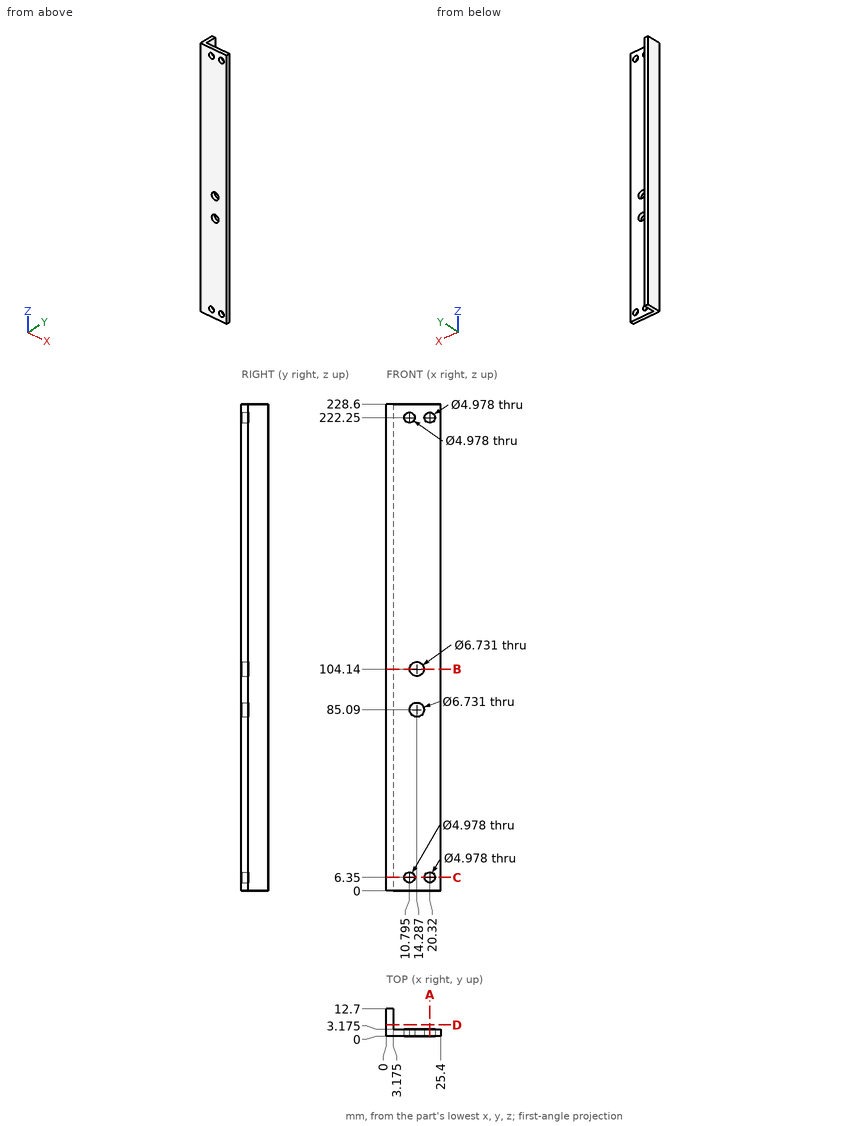
Input: dimensioned drawing with shaded views. Units: mm. Origin: part minimum x, y, z. Coordinates: 2 decimals unless noted, no trailing zeros. Order: outer loops, then holes, each group sorted by start corner. A loop starts at its lowest first (then second) coordinate and runs counter-clockwise, first axis right, second up.
Item 1: Material intervals for line 1 along X through (y, z) = (1.45, 222.25) (1 decimal); line 2 along Z through (x, y) = (20.32, 1.6); line 3 along X through (y, z) = (1.35, 104.14), sorted ascending.
Answer:
line 1: x = 0 to 8.3, 13.3 to 17.8, 22.8 to 25.4
line 2: z = 0 to 3.86, 8.84 to 219.76, 224.74 to 228.6
line 3: x = 0 to 10.92, 17.65 to 25.4
Item 2: Contact query for flat-ended pins moving along their axis: P1, Ø4, axis at x = 10.795, z = 6.35, coming from the +Y side; P2, Ø5, axis at y = 6, z = 109, coming from the +X side (1 decimal); P3, Ø11, axis at x = 14.29, z = 104.14, coming from the +Y side (1 decimal). Output: stop coordinate, or through.
Answer:
P1: passes through
P2: stops at x = 3.2
P3: stops at y = 3.2
Item 3: Section query A-A (x = 20.32). Output: boundary loops of the cut face in (y, z) (1 decimal).
Answer:
outline: (0, 0) - (3.2, 0) - (3.2, 3.9) - (0, 3.9) - close; (0, 8.8) - (3.2, 8.8) - (3.2, 219.8) - (0, 219.8) - close; (0, 224.7) - (3.2, 224.7) - (3.2, 228.6) - (0, 228.6) - close
Item 4: Section query C-C (z = 6.35). Output: boundary loops of the cut face in (x, y) (1 decimal).
Answer:
outline: (0, 0) - (8.3, 0) - (8.3, 3.2) - (3.2, 3.2) - (3.2, 12.7) - (0, 12.7) - close; (13.3, 0) - (17.8, 0) - (17.8, 3.2) - (13.3, 3.2) - close; (22.8, 0) - (25.4, 0) - (25.4, 3.2) - (22.8, 3.2) - close
Item 5: Section query D-D (y = 5.25). Output: boundary loops of the cut face in (x, z) (1 decimal).
Answer:
outline: (0, 0) - (3.2, 0) - (3.2, 228.6) - (0, 228.6) - close
Item 6: Section query B-B (z = 104.14). Output: boundary loops of the cut face in (x, y) (1 decimal).
Answer:
outline: (0, 0) - (10.9, 0) - (10.9, 3.2) - (3.2, 3.2) - (3.2, 12.7) - (0, 12.7) - close; (17.7, 0) - (25.4, 0) - (25.4, 3.2) - (17.7, 3.2) - close
